from build123d import *

# Parameters (mm, degrees)
ESQUISSE3_W                  = 5.995341806
ESQUISSE3_H                  = 6
ESQUISSE4_W                  = 15.004658194
ESQUISSE4_H                  = 3
ESQUISSE5_W                  = 5
ESQUISSE5_H                  = 1
ENL_V_MAT_EXTRU_1_DEPTH      = 12
CHANFREIN1_SIZE              = 0.5
ESQUISSE6_W                  = 3
ESQUISSE6_H                  = 3
ESQUISSE7_W                  = 1.2
ESQUISSE7_H                  = 16.4
ESQUISSE8_W                  = 9.3
ESQUISSE8_H                  = 7.5
R_P_TITION_CIRCULAIRE1_COUNT = 6
CONG_1_R                     = 1
CHANFREIN2_SIZE              = 0.5


with BuildPart() as part:
    # Esquisse1 → Révolution1 (revolve)
    with BuildSketch(Plane(origin=(0, 0, 0), x_dir=(0, 0, -1), z_dir=(1, 0, 0))):
        Polygon((0, 0), (0, 16.4), (-23, 16.4), (-23, 18.5), (-44.5, 18.5), (-44.5, 0), align=None)
    revolve(axis=Axis((0, 0, 44.5), (0, 0, -1)))

    # Esquisse3 → Révolution2 (revolve)
    with BuildSketch(Plane(origin=(0, 0, 0), x_dir=(0, 0, -1), z_dir=(1, 0, 0))):
        with Locations((-47.497670903, 11.5)):
            Rectangle(ESQUISSE3_W, ESQUISSE3_H)
    revolve(axis=Axis((0, 8.5, 50.495341806), (0, 0, -1)))

    # Esquisse4 → Révolution3 (revolve)
    with BuildSketch(Plane(origin=(0, 0, 0), x_dir=(0, 0, -1), z_dir=(1, 0, 0))):
        with Locations((-57.997670903, 10)):
            Rectangle(ESQUISSE4_W, ESQUISSE4_H)
    revolve(axis=Axis((0, 8.5, 50.495341806), (0, 0, 1)))

    # Esquisse5 → Enlèv. mat.-Extru.1 (cut)
    with BuildSketch(Plane.XY.offset(65.5)):
        with Locations((0, 11.4)):
            Rectangle(ESQUISSE5_W, ESQUISSE5_H)
    extrude(amount=-ENL_V_MAT_EXTRU_1_DEPTH, mode=Mode.SUBTRACT)

    # Chanfrein1
    chanfrein1_edges = [part.edges().sort_by_distance(p)[0] for p in [
        (0, 5.5, 65.5),
        (0, 10.9, 53.5),
    ]]
    chamfer(chanfrein1_edges, length=CHANFREIN1_SIZE)

    # Esquisse6 → Révolution4 (revolve)
    with BuildSketch(Plane(origin=(0, 0, 0), x_dir=(0, 0, -1), z_dir=(1, 0, 0))):
        with Locations((1.5, 1.5)):
            Rectangle(ESQUISSE6_W, ESQUISSE6_H)
    revolve(axis=Axis((0, 0, 0), (0, 0, -1)))

    # Esquisse7 → Révolution5 (revolve)
    with BuildSketch(Plane(origin=(0, 0, 0), x_dir=(0, 0, -1), z_dir=(1, 0, 0))):
        with Locations((3.6, 8.2)):
            Rectangle(ESQUISSE7_W, ESQUISSE7_H)
    revolve(axis=Axis((0, 0, -3), (0, 0, -1)))

    # Esquisse8 → Révolution6 (revolve)
    with BuildSketch(Plane(origin=(0, 0, 0), x_dir=(0, 0, -1), z_dir=(1, 0, 0))):
        with Locations((8.85, 3.75)):
            Rectangle(ESQUISSE8_W, ESQUISSE8_H)
    revolve(axis=Axis((0, 0, -4.2), (0, 0, -1)))

    # Esquisse12 → Dégagement M31 (revolve, cut)
    with BuildSketch(Plane(origin=(15.5, 0, 44.5), x_dir=(0, -1, 0), z_dir=(1, 0, 0))):
        Polygon((0, 0), (0, 11.021463052), (1.7, 10), (1.7, 0), align=None)
    d_gagement_m31 = revolve(axis=Axis((15.5, 0, 50.85), (0, 0, -1)), mode=Mode.SUBTRACT)

    # Répétition circulaire1: Dégagement M31 ×6 about axis
    r_p_tition_circulaire1_axis = Axis((0, 0, 0), (0, 0, 1))
    for i in range(1, R_P_TITION_CIRCULAIRE1_COUNT):
        add(d_gagement_m31.rotate(r_p_tition_circulaire1_axis, i * 360 / R_P_TITION_CIRCULAIRE1_COUNT), mode=Mode.SUBTRACT)

    # Congé1
    cong_1_edges = [part.edges().sort_by_distance(p)[0] for p in [
        (0, -16.4, 0),
    ]]
    fillet(cong_1_edges, radius=CONG_1_R)

    # Chanfrein2
    chanfrein2_edges = [part.edges().sort_by_distance(p)[0] for p in [
        (0, 2.5, 50.495341806),
    ]]
    chamfer(chanfrein2_edges, length=CHANFREIN2_SIZE)


solid = part.part
Build history of the part. All positions in model axes, mm. A direction names the side the tool comes from. Coordinates: 2 decimals unless noted, no trailing zeros. Write each loop counter-clockwise with the first axis right and the second up, starting at its lowest first coordinate (ties: lowest second). Pieces come first, ordered by that corner, then holes.
(1) 3-axis set-ups, long thin cutter, end or side, ignore diameter. For faces 1 (the cylindrical face through (-18.06, -4.01, 33.9)), 2 (the flat face through (-3.4, -7.1, -4.2)), 3 (the cylindrical face through (-6.72, -12.07, 39.57)): which of +Z, -Z, +X, -X, +Y, -Y reach the whole face in a straight line?
(2) Drill centre lines: line 1 (Z direction, x = -13, y = -2.5); line 2 (Z direction, x = -0.5, y = -6.5); line 3 (Y direction, x = -7, z = 39). Where is each one in solid material? Low to high.
(3) Pin check, flat tips, straight feed: pin 1 Ø2 at (x, z) = (10, 28.5) entering from -Y; pin 2 Ø4 at (x, y) = (-7.75, -13.42) entering from +Z; pin 3 Ø4 at (x, y) = (-15.5, 0) entering from -Z. Stop position of each tip, or through.
(4) Mould opens along Y. For faces 4 (the cylindrical face through (16.26, -2.13, 12.15)), 5 (the conical face through (-8.043, 13.462, 33.656)), 6 (the flat face through (0, 0, -13.5)) say: pulls with the +Y half, pulls with the -Y half, needs draft (parallel to the pull), parting line crosses it, or undercut.
(5) Cut at A-A on z = 41. List the corners of the cut face in (x, y).
(6) Cut at B-B on z = 31. List the corners of the cut face in (x, y).
Working result:
1. face 1: +Z, -Z
1. face 2: -Z
1. face 3: +Z
2. line 1: z = -4.2 to -3, 0 to 44.5
2. line 2: z = -13.5 to -3, 0 to 44.5
2. line 3: y = -17.12 to -14.95, -11.9 to 11.9, 14.95 to 17.12
3. pin 1: stops at y = -16.16
3. pin 2: stops at z = 44.5
3. pin 3: stops at z = -4.2
4. face 4: parting line crosses it
4. face 5: undercut
4. face 6: needs draft
5. outline: circle Ø37 at (0, 0); hole circle Ø3.4 at (-15.5, 0); hole circle Ø3.4 at (-7.75, -13.42); hole circle Ø3.4 at (-7.75, 13.42); hole circle Ø3.4 at (7.75, -13.42); hole circle Ø3.4 at (7.75, 13.42); hole circle Ø3.4 at (15.5, 0)
6. outline: circle Ø37 at (0, 0)
